Part model, mm, in its own coordinate system. A direction names the side the tool comes from. Round coordinates to 2 decimals unless told otherwise and drop trailing zeros. Loops run counter-clockwise (first coordinate to the right, second up) from the corner with the lowest first, then second, coordinate; pieces in that order, holes last.
from build123d import *

# Parameters (mm, degrees)
SKETCH1_R           = 5.875
SKETCH1_R_2         = 1.7
BOSS_EXTRUDE1_DEPTH = 1.25
SKETCH2_R           = 14.935
SKETCH2_R_2         = 1.7
SKETCH2_R_3         = 3.220003918
BOSS_EXTRUDE2_DEPTH = 5


with BuildPart() as part:
    # Sketch1 → Boss-Extrude1 (new body)
    with BuildSketch(Plane.XY):
        with Locations((19.5, 0)):
            Circle(SKETCH1_R)
        with Locations((19.5, 0)):
            Circle(SKETCH1_R_2, mode=Mode.SUBTRACT)
    extrude(amount=-BOSS_EXTRUDE1_DEPTH)

    # Sketch2 → Boss-Extrude2 (add)
    with BuildSketch(Plane(origin=(0, 0, -1.25), x_dir=(-1, 0, 0), z_dir=(0, 0, -1))):
        with Locations((-19.5, 0)):
            Circle(SKETCH2_R)
        with Locations((-19.5, -11.235)):
            Circle(SKETCH2_R_2, mode=Mode.SUBTRACT)
        with Locations((-19.5, 0)):
            Circle(SKETCH2_R_3, mode=Mode.SUBTRACT)
        with Locations((-27.444344687, -7.944344687)):
            Circle(SKETCH2_R_2, mode=Mode.SUBTRACT)
        with Locations((-30.735, 0)):
            Circle(SKETCH2_R_2, mode=Mode.SUBTRACT)
        with Locations((-27.444344687, 7.944344686)):
            Circle(SKETCH2_R_2, mode=Mode.SUBTRACT)
        with Locations((-19.5, 11.235)):
            Circle(SKETCH2_R_2, mode=Mode.SUBTRACT)
        with Locations((-11.555655313, 7.944344686)):
            Circle(SKETCH2_R_2, mode=Mode.SUBTRACT)
        with Locations((-8.265, 0)):
            Circle(SKETCH2_R_2, mode=Mode.SUBTRACT)
        with Locations((-11.555655313, -7.944344687)):
            Circle(SKETCH2_R_2, mode=Mode.SUBTRACT)
    extrude(amount=BOSS_EXTRUDE2_DEPTH)


solid = part.part
1) Slice it at C-C, the plane y = 8.5. Give the cut face in (x, z), then the cut area to 3 significant figures.
Values:
outline: (7.22, -6.25) - (9.95, -6.25) - (9.95, -1.25) - (7.22, -1.25) - close; (13.16, -6.25) - (25.84, -6.25) - (25.84, -1.25) - (13.16, -1.25) - close; (29.05, -6.25) - (31.78, -6.25) - (31.78, -1.25) - (29.05, -1.25) - close
area: 90.7 mm2
2) Wall check: line 1 along Y through (x, z) = (19.5, -2.75) (3 decimals); line 2 along Y through (x, z) = (11, -6); line 3 along X through (y, z) = (7, -2). Give the ranges that are in metal, low to high.
Values:
line 1: y = -14.935 to -12.935, -9.535 to -3.22, 3.22 to 9.535, 12.935 to 14.935
line 2: y = -12.28 to -9.55, -6.34 to 6.34, 9.55 to 12.28
line 3: x = 6.31 to 10.14, 12.97 to 26.03, 28.86 to 32.69
3) Slice it at D-D, the plane x = 11.5. Give the cut face in (y, z), then the cut area to 3 significant figures.
Values:
outline: (-12.61, -6.25) - (-9.64, -6.25) - (-9.64, -1.25) - (-12.61, -1.25) - close; (-6.25, -6.25) - (6.25, -6.25) - (6.25, -1.25) - (-6.25, -1.25) - close; (9.64, -6.25) - (12.61, -6.25) - (12.61, -1.25) - (9.64, -1.25) - close
area: 92.1 mm2
4) Slice it at B-B, the plane x = 19.5. Give the cut face in (y, z) (3 decimals), then the cut area to 3 significant figures.
Values:
outline: (-14.935, -6.25) - (-12.935, -6.25) - (-12.935, -1.25) - (-14.935, -1.25) - close; (-9.535, -6.25) - (-3.22, -6.25) - (-3.22, -1.25) - (-1.7, -1.25) - (-1.7, 0) - (-5.875, 0) - (-5.875, -1.25) - (-9.535, -1.25) - close; (1.7, -1.25) - (3.22, -1.25) - (3.22, -6.25) - (9.535, -6.25) - (9.535, -1.25) - (5.875, -1.25) - (5.875, 0) - (1.7, 0) - close; (12.935, -6.25) - (14.935, -6.25) - (14.935, -1.25) - (12.935, -1.25) - close
area: 93.6 mm2
5) Mould opens along Z. For faces 4 (the face through (31.35, -9.09, -3.72)), 5 (the face through (20.9, -1.4, -1.25)), 6 (the face through (19.7, -6.4, -1.25)) say: released by +Z, released by -Z, zero draft, split by the parting line, or undercut.
Values:
face 4: zero draft
face 5: released by -Z
face 6: released by +Z
6) Slice it at A-A, the plane y = 0. Give the cut face in (x, z) (3 decimals).
Values:
outline: (4.565, -6.25) - (6.565, -6.25) - (6.565, -1.25) - (4.565, -1.25) - close; (9.965, -6.25) - (16.28, -6.25) - (16.28, -1.25) - (17.8, -1.25) - (17.8, 0) - (13.625, 0) - (13.625, -1.25) - (9.965, -1.25) - close; (21.2, -1.25) - (22.72, -1.25) - (22.72, -6.25) - (29.035, -6.25) - (29.035, -1.25) - (25.375, -1.25) - (25.375, 0) - (21.2, 0) - close; (32.435, -6.25) - (34.435, -6.25) - (34.435, -1.25) - (32.435, -1.25) - close
7) Tool access for faces 1 (the face through (13.63, 0.26, -0.62)), 2 (the face through (22.717, 0.142, -3.715)), 3 (the face through (25.823, -7.434, -3.715)): list every direction of +Z, -Z, +X, -X, +Y, -Y with a clear straight run to the whole face (end or side of a thin tool).
Values:
face 1: +Z
face 2: -Z
face 3: +Z, -Z
8) Drop flat-ended pins along their axis: pin 1 Ø2 at (x, y) = (27.44, -7.94) entering from +Z; pin 2 Ø1.5 at (x, z) = (27.5, -1.5) entering from -Y; pin 3 Ø1.5 at (x, z) = (12, -5.5) entering from +Y; pin 4 Ø4 at (x, y) = (11.56, 7.94) entering from +Z. Give the stop position or say it passes through.
Values:
pin 1: passes through
pin 2: stops at y = -13.06
pin 3: stops at y = 13.32
pin 4: stops at z = -1.25
